from build123d import *

# Parameters (mm, degrees)
F0_W     = 28
F0_H     = 22
F1_DEPTH = 15
F3_R     = 1.5
F5_D     = 1.5
F6_D     = 1.5
F7_D     = 1.5
F8_D     = 1.5
F2_W     = 16
F2_H     = 4
F9_DEPTH = 10


with BuildPart() as f1:
    # F0 (on Top) → F1 (new body)
    with BuildSketch(Plane.XY):
        with Locations((-1.261453, -0.651873)):
            Rectangle(F0_W, F0_H)
        Polygon((-11.761453, -10.151873), (-11.761453, 8.848127), (5.738547, 8.848127), (9.238547, 8.848127), (9.238547, -10.151873), (5.738547, -10.151873), align=None, mode=Mode.SUBTRACT)
    extrude(amount=F1_DEPTH)

    # F3
    f3_edges = [f1.edges().sort_by_distance(p)[0] for p in [
        (12.738547, 10.348127, 7.5),
        (12.738547, -11.651873, 7.5),
        (-15.261453, -11.651873, 7.5),
        (-15.261453, 10.348127, 7.5),
    ]]
    fillet(f3_edges, radius=F3_R)

    # F5 (through all)
    with Locations(Plane.XY.offset(15)):
        with Locations((-13.011453, 4.098127)):
            Hole(F5_D / 2)

    # F6 (through all)
    with Locations(Plane.XY.offset(15)):
        with Locations((-13.011453, -5.401873)):
            Hole(F6_D / 2)

    # F7 (through all)
    with Locations(Plane.XY.offset(15)):
        with Locations((10.488547, -5.401873)):
            Hole(F7_D / 2)

    # F8 (through all)
    with Locations(Plane.XY.offset(15)):
        with Locations((10.488547, 4.098127)):
            Hole(F8_D / 2)

    # F2 (on face) → F9 (cut)
    with BuildSketch(Plane.YZ.offset(12.738547)):
        with Locations((-0.651873, 2)):
            Rectangle(F2_W, F2_H)
    extrude(amount=-F9_DEPTH, mode=Mode.SUBTRACT)


solid = f1.part
Could you check a few things on this model? Use its own coordinates, in mm. A direction names the side the tool comes from. Give positions to 0.01 mm unless a question says otherwise; leave off trailing zeros. Order: outer loops, then holes, each group sorted by start corner. A loop starts at its lowest first (then second) coordinate and runs counter-clockwise, first axis right, second up. Notation, with made-up numbers: (-14.75, -14.5) - (10.25, -14.5) arc R17 ccw to (10.25, -7.5) - close; hole circle Ø1 at (31, 54). An arc over 180 degrees is marked (long way). Return JSON: item names as keys, results as strings. Group by question number.
Q1. Suppose I cut it at D-D, the plane x = 10.75. Please give me the cut outline in (y, z), and give its area (3 significant figures).
Q2. Which directions (+Z, -Z, +X, -X, +Y, -Y) give clear straight access to the entire face, cutting with the end or side of a thin tool? Please do faces 1 (the face through (-13, -1, 0)), 2 (the face through (-1, 8.848, 7)), 3 (the face through (11, 7.348, 2)).
Q3. Suppose I cut it at C-C, the plane z = 2.5. Please give me the cut outline in (x, y), and give its area (3 significant figures).
Q4. Thinking about a two-plate mould opening in X: for faces 4 (the face through (-15, -11, 8)), 5 (the face through (11, -1, 4)), 6 (the face through (-11.761, -1, 7)), which applies, pulls with the +X half, pulls with the -X half, needs draft (parallel to the pull), parting line crosses it, or undercut?
Q5. Suppose I cut it at A-A, the plane y = 8. Please give me the cut outline in (x, z).
Q6. Will these pins go through, and if not, where does the flat tip stop? pin 1 Ø1.4 at (x, y) = (-13.01, 4.1) entering from +Z; pin 2 Ø1.7 at (x, y) = (10.49, 4.1) entering from -Z.
Q7. Suppose I cut it at B-B, the plane x = -8.5. Please give me the cut outline in (y, z), and give its area (3 significant figures).
Q8. Please list where these lines run through material, in increasing order: line 1 along Y through (x, z) = (10.5, 14); line 2 along X through (y, z) = (4, 12.75) (3 decimals); line 3 along X through (y, z) = (-9, 7.75). Write a range as [from, to].
Resolved:
{
 "1": {"outline": "(-11.65, 0) - (-8.65, 0) - (-8.65, 4) - (-6.1, 4) - (-6.1, 15) - (-11.65, 15) - close; (-4.7, 4) - (3.4, 4) - (3.4, 15) - (-4.7, 15) - close; (4.8, 4) - (7.35, 4) - (7.35, 0) - (10.35, 0) - (10.35, 15) - (4.8, 15) - close", "area": "235 mm2"},
 "2": {"face 1": "-Z, +X, -X, +Y, -Y", "face 2": "+Z, -Z", "face 3": "-Z, +X"},
 "3": {"outline": "(-15.26, -10.15) arc R1.5 ccw to (-13.76, -11.65) - (11.24, -11.65) arc R1.5 ccw to (12.74, -10.15) - (12.74, -8.65) - (9.24, -8.65) - (9.24, -10.15) - (-11.76, -10.15) - (-11.76, 8.85) - (9.24, 8.85) - (9.24, 7.35) - (12.74, 7.35) - (12.74, 8.85) arc R1.5 ccw to (11.24, 10.35) - (-13.76, 10.35) arc R1.5 ccw to (-15.26, 8.85) - close; hole circle Ø1.5 at (-13.01, -5.4); hole circle Ø1.5 at (-13.01, 4.1)", "area": "156 mm2"},
 "4": {"face 4": "pulls with the -X half", "face 5": "needs draft", "face 6": "undercut"},
 "5": {"outline": "(-15.26, 0) - (-11.76, 0) - (-11.76, 15) - (-15.26, 15) - close; (9.24, 0) - (12.74, 0) - (12.74, 15) - (9.24, 15) - close"},
 "6": {"pin 1": "passes through", "pin 2": "stops at z = 4"},
 "7": {"outline": "(-11.65, 0) - (-10.15, 0) - (-10.15, 15) - (-11.65, 15) - close; (8.85, 0) - (10.35, 0) - (10.35, 15) - (8.85, 15) - close", "area": "45.0 mm2"},
 "8": {"line 1": "y = [-11.65, -6.15], [-4.65, 3.35], [4.85, 10.35]", "line 2": "x = [-15.261, -13.755], [-12.268, -11.761], [9.239, 9.745], [11.232, 12.739]", "line 3": "x = [-15.26, -11.76], [9.24, 12.74]"}
}
